```python
from build123d import *

# Parameters (mm, degrees)
SKETCH1_W              = 44
SKETCH1_H              = 26
BOSS_EXTRUDE1_DEPTH    = 1.45
SKETCH3_R              = 4
CUT_EXTRUDE1_DEPTH     = 52.128294515
SKETCH4_R              = 1
CUT_EXTRUDE2_DEPTH     = 52.128294515
CIRPATTERN1_COUNT      = 8
SKETCH7_R              = 1.25
CUT_EXTRUDE3_DEPTH     = 52.128294515
CIRPATTERN2_COUNT      = 8
SKETCH9_R              = 1.25
CUT_EXTRUDE4_DEPTH     = 52.128294515
CIRPATTERN3_COUNT      = 4
SKETCH10_R             = 1.25
CUT_EXTRUDE5_DEPTH     = 52.128294515
SKETCH11_R             = 1.25
CUT_EXTRUDE6_DEPTH     = 52.128294515
SKETCH14_W             = 4.5
SKETCH14_H             = 8
CUT_EXTRUDE7_DEPTH     = 52.128294515
FILLET1_R              = 1
FILLET1_OF_MIRROR2_R   = 1
SKETCH16_W             = 1.45
SKETCH16_H             = 26
BOSS_EXTRUDE4_DEPTH    = 31.05
SKETCH21_W             = 5
SKETCH21_H             = 8
CUT_EXTRUDE10_DEPTH    = 60.521025697
SKETCH22_R             = 4
CUT_EXTRUDE11_DEPTH    = 60.521025697
SKETCH23_R             = 1
CUT_EXTRUDE12_DEPTH    = 60.521025697
CIRPATTERN5_COUNT      = 8
SKETCH24_W             = 31.05
SKETCH24_H             = 2
CUT_EXTRUDE13_DEPTH    = 60.521025697
SKETCH26_W             = 31.05
SKETCH26_H             = 2
CUT_EXTRUDE14_DEPTH    = 60.521025697
FILLET3_R              = 2
SKETCH28_R             = 1
CUT_EXTRUDE16_DEPTH    = 10
SKETCH30_R             = 1
CUT_EXTRUDE17_DEPTH    = 10
SKETCH31_W             = 4
SKETCH31_H             = 10
CUT_EXTRUDE18_DEPTH    = 3
FILLET4_R              = 1
LPATTERN1_COUNT        = 2
LPATTERN1_PITCH        = 8
FILLET4_OF_LPATTERN1_R = 1
MIRROR3_START          = 42.55
MIRROR3_OUTLINE_R      = 1
MIRROR3_DEPTH          = 1.45
SKETCH34_W             = 39
SKETCH34_H             = 1.45
BOSS_EXTRUDE8_DEPTH    = 3.35
SKETCH37_W             = 2.5
SKETCH37_H             = 2
CUT_EXTRUDE20_DEPTH    = 3.35
SKETCH35_W             = 2.5
SKETCH35_H             = 2
CUT_EXTRUDE21_DEPTH    = 3.35
FILLET5_R              = 1.5
FILLET6_R              = 2
FILLET7_R              = 1.5
FILLET8_R              = 1.5
FILLET9_R              = 2


# Read off the part's stored shape, not the designer's step: Mirror3
with BuildPart() as part:
    # Sketch1 → Boss-Extrude1 (new body)
    with BuildSketch(Plane.XY):
        with Locations((22, 13)):
            Rectangle(SKETCH1_W, SKETCH1_H)
    extrude(amount=BOSS_EXTRUDE1_DEPTH)

    # Sketch3 → Cut-Extrude1 (cut, through all)
    with BuildSketch(Plane.XY.offset(1.45)):
        with Locations((22, 13)):
            Circle(SKETCH3_R)
    extrude(amount=-CUT_EXTRUDE1_DEPTH, mode=Mode.SUBTRACT)

    # Sketch4 → Cut-Extrude2 (cut, through all)
    with BuildSketch(Plane.XY.offset(1.45)):
        with Locations((22, 21)):
            Circle(SKETCH4_R)
    cut_extrude2 = extrude(amount=-CUT_EXTRUDE2_DEPTH, mode=Mode.SUBTRACT)

    # CirPattern1: Cut-Extrude2 ×8 about axis
    cirpattern1_axis = Axis((22, 13, 0), (0, 0, 1))
    for i in range(1, CIRPATTERN1_COUNT):
        add(cut_extrude2.rotate(cirpattern1_axis, i * 360 / CIRPATTERN1_COUNT), mode=Mode.SUBTRACT)

    # Sketch7 → Cut-Extrude3 (cut, through all)
    with BuildSketch(Plane.XY.offset(1.45)):
        with Locations((25.322496408, 21)):
            Circle(SKETCH7_R)
    cut_extrude3 = extrude(amount=-CUT_EXTRUDE3_DEPTH, mode=Mode.SUBTRACT)

    # CirPattern2: Cut-Extrude3 ×8 about axis
    cirpattern2_axis = Axis((22, 13, 0), (0, 0, 1))
    for i in range(1, CIRPATTERN2_COUNT):
        add(cut_extrude3.rotate(cirpattern2_axis, i * 360 / CIRPATTERN2_COUNT), mode=Mode.SUBTRACT)

    # Sketch9 → Cut-Extrude4 (cut, through all)
    with BuildSketch(Plane.XY.offset(1.45)):
        with Locations((30, 21)):
            Circle(SKETCH9_R)
    cut_extrude4 = extrude(amount=-CUT_EXTRUDE4_DEPTH, mode=Mode.SUBTRACT)

    # CirPattern3: Cut-Extrude4 ×4 about axis
    cirpattern3_axis = Axis((22, 13, 0), (0, 0, 1))
    for i in range(1, CIRPATTERN3_COUNT):
        add(cut_extrude4.rotate(cirpattern3_axis, i * 360 / CIRPATTERN3_COUNT), mode=Mode.SUBTRACT)

    # Sketch10 → Cut-Extrude5 (cut, through all)
    with BuildSketch(Plane.XY.offset(1.45)):
        with Locations((39.5, 21)):
            Circle(SKETCH10_R)
    cut_extrude5 = extrude(amount=-CUT_EXTRUDE5_DEPTH, mode=Mode.SUBTRACT)

    # Sketch11 → Cut-Extrude6 (cut, through all)
    with BuildSketch(Plane.XY.offset(1.45)):
        with Locations((39.5, 5)):
            Circle(SKETCH11_R)
    cut_extrude6 = extrude(amount=-CUT_EXTRUDE6_DEPTH, mode=Mode.SUBTRACT)

    # Mirror1: Cut-Extrude5, Cut-Extrude6 across plane
    add(cut_extrude5.mirror(Plane(origin=(22, 0, 0), x_dir=(0, 0, 1), z_dir=(1, 0, 0))), mode=Mode.SUBTRACT)
    add(cut_extrude6.mirror(Plane(origin=(22, 0, 0), x_dir=(0, 0, 1), z_dir=(1, 0, 0))), mode=Mode.SUBTRACT)

    # Sketch14 → Cut-Extrude7 (cut, through all)
    with BuildSketch(Plane.XY.offset(1.45)):
        with Locations((8.25, 13)):
            Rectangle(SKETCH14_W, SKETCH14_H)
    cut_extrude7 = extrude(amount=-CUT_EXTRUDE7_DEPTH, mode=Mode.SUBTRACT)

    # Fillet1
    fillet1_edges = [part.edges().sort_by_distance(p)[0] for p in [
        (10.5, 9, 0.725),
        (6, 9, 0.725),
        (6, 17, 0.725),
        (10.5, 17, 0.725),
    ]]
    fillet(fillet1_edges, radius=FILLET1_R)

    # Mirror2: Cut-Extrude7 across plane
    add(cut_extrude7.mirror(Plane(origin=(22, 0, 0), x_dir=(0, 0, 1), z_dir=(1, 0, 0))), mode=Mode.SUBTRACT)

    # Fillet1 of Mirror2
    fillet1_of_mirror2_edges = [part.edges().sort_by_distance(p)[0] for p in [
        (33.5, 9, 0.725),
        (38, 9, 0.725),
        (38, 17, 0.725),
        (33.5, 17, 0.725),
    ]]
    fillet(fillet1_of_mirror2_edges, radius=FILLET1_OF_MIRROR2_R)

    # Sketch16 → Boss-Extrude4 (add)
    with BuildSketch(Plane.XY.offset(1.45)):
        with Locations((0.725, 13)):
            Rectangle(SKETCH16_W, SKETCH16_H)
    extrude(amount=BOSS_EXTRUDE4_DEPTH)

    # Sketch21 → Cut-Extrude10 (cut, through all)
    with BuildSketch(Plane(origin=(1.45, 0, 0), x_dir=(0, 0, -1), z_dir=(1, 0, 0))):
        with Locations((-32.5, 13)):
            Rectangle(SKETCH21_W, SKETCH21_H)
    extrude(amount=-CUT_EXTRUDE10_DEPTH, mode=Mode.SUBTRACT)

    # Sketch22 → Cut-Extrude11 (cut, through all)
    with BuildSketch(Plane(origin=(1.45, 0, 0), x_dir=(0, 0, -1), z_dir=(1, 0, 0))):
        with Locations((-30, 13)):
            Circle(SKETCH22_R)
    extrude(amount=-CUT_EXTRUDE11_DEPTH, mode=Mode.SUBTRACT)

    # Sketch23 → Cut-Extrude12 (cut, through all)
    with BuildSketch(Plane(origin=(1.45, 0, 0), x_dir=(0, 0, -1), z_dir=(1, 0, 0))):
        with Locations((-22, 13)):
            Circle(SKETCH23_R)
    cut_extrude12 = extrude(amount=-CUT_EXTRUDE12_DEPTH, mode=Mode.SUBTRACT)

    # CirPattern5: Cut-Extrude12 ×8 about axis, 2 skipped
    cirpattern5_axis = Axis((0, 13, 30), (1, 0, 0))
    add([cut_extrude12.rotate(cirpattern5_axis, i * 360 / CIRPATTERN5_COUNT) for i in range(1, CIRPATTERN5_COUNT) if i not in (4, 5)], mode=Mode.SUBTRACT)

    # Sketch24 → Cut-Extrude13 (cut, through all)
    with BuildSketch(Plane(origin=(1.45, 0, 0), x_dir=(0, 0, -1), z_dir=(1, 0, 0))):
        with Locations((-16.975, 25)):
            Rectangle(SKETCH24_W, SKETCH24_H)
    extrude(amount=-CUT_EXTRUDE13_DEPTH, mode=Mode.SUBTRACT)

    # Sketch26 → Cut-Extrude14 (cut, through all)
    with BuildSketch(Plane(origin=(1.45, 0, 0), x_dir=(0, 0, -1), z_dir=(1, 0, 0))):
        with Locations((-16.975, 1)):
            Rectangle(SKETCH26_W, SKETCH26_H)
    extrude(amount=-CUT_EXTRUDE14_DEPTH, mode=Mode.SUBTRACT)

    # Fillet3
    fillet3_edges = [part.edges().sort_by_distance(p)[0] for p in [
        (0.725, 17, 32.5),
        (0.725, 9, 32.5),
        (0.725, 24, 32.5),
        (0.725, 2, 32.5),
    ]]
    fillet(fillet3_edges, radius=FILLET3_R)

    # Sketch28 → Cut-Extrude16 (cut)
    with BuildSketch(Plane.ZY):
        with Locations((12, 21)):
            Circle(SKETCH28_R)
    extrude(amount=-CUT_EXTRUDE16_DEPTH, mode=Mode.SUBTRACT)

    # Sketch30 → Cut-Extrude17 (cut)
    with BuildSketch(Plane.ZY):
        with Locations((12, 5)):
            Circle(SKETCH30_R)
    extrude(amount=-CUT_EXTRUDE17_DEPTH, mode=Mode.SUBTRACT)

    # Sketch31 → Cut-Extrude18 (cut)
    with BuildSketch(Plane.ZY):
        with Locations((16, 13)):
            Rectangle(SKETCH31_W, SKETCH31_H)
    cut_extrude18 = extrude(amount=-CUT_EXTRUDE18_DEPTH, mode=Mode.SUBTRACT)

    # Fillet4
    fillet4_edges = [part.edges().sort_by_distance(p)[0] for p in [
        (0.725, 8, 14),
        (0.725, 18, 14),
        (0.725, 18, 18),
        (0.725, 8, 18),
    ]]
    fillet(fillet4_edges, radius=FILLET4_R)

    # LPattern1: Cut-Extrude18 ×2
    with Locations(*[(0, 0, -i * LPATTERN1_PITCH) for i in range(1, LPATTERN1_COUNT)]):
        add(cut_extrude18, mode=Mode.SUBTRACT)

    # Fillet4 of LPattern1
    fillet4_of_lpattern1_edges = [part.edges().sort_by_distance(p)[0] for p in [
        (0.725, 8, 6),
        (0.725, 18, 6),
        (0.725, 18, 10),
        (0.725, 8, 10),
    ]]
    fillet(fillet4_of_lpattern1_edges, radius=FILLET4_OF_LPATTERN1_R)

    # Mirror3 outline → Mirror3 (add)
    with BuildSketch(Plane.YZ.offset(MIRROR3_START)):
        with BuildLine():
            Line((7, 32.5), (4, 32.5))
            ThreePointArc((4, 32.5), (2.585786438, 31.914213562), (2, 30.5))
            Line((2, 30.5), (2, 1.45))
            Line((2, 1.45), (24, 1.45))
            Line((24, 1.45), (24, 30.5))
            ThreePointArc((24, 30.5), (23.414213562, 31.914213562), (22, 32.5))
            Line((22, 32.5), (19, 32.5))
            ThreePointArc((19, 32.5), (17.585786438, 31.914213562), (17, 30.5))
            Line((17, 30.5), (17, 30))
            ThreePointArc((17, 30), (13, 26), (9, 30))
            Line((9, 30), (9, 30.5))
            ThreePointArc((9, 30.5), (8.414213562, 31.914213562), (7, 32.5))
        make_face()
        with Locations((5, 12)):
            Circle(MIRROR3_OUTLINE_R, mode=Mode.SUBTRACT)
        with BuildLine():
            Line((18, 9), (18, 7))
            ThreePointArc((18, 7), (17.707106781, 6.292893219), (17, 6))
            Line((17, 6), (9, 6))
            ThreePointArc((9, 6), (8.292893219, 6.292893219), (8, 7))
            Line((8, 7), (8, 9))
            ThreePointArc((8, 9), (8.292893219, 9.707106781), (9, 10))
            Line((9, 10), (17, 10))
            ThreePointArc((17, 10), (17.707106781, 9.707106781), (18, 9))
        make_face(mode=Mode.SUBTRACT)
        with BuildLine():
            ThreePointArc((18, 15), (17.707106781, 14.292893219), (17, 14))
            Line((17, 14), (9, 14))
            ThreePointArc((9, 14), (8.292893219, 14.292893219), (8, 15))
            Line((8, 15), (8, 17))
            ThreePointArc((8, 17), (8.292893219, 17.707106781), (9, 18))
            Line((9, 18), (17, 18))
            ThreePointArc((17, 18), (17.707106781, 17.707106781), (18, 17))
            Line((18, 17), (18, 15))
        make_face(mode=Mode.SUBTRACT)
        with Locations((21, 12)):
            Circle(MIRROR3_OUTLINE_R, mode=Mode.SUBTRACT)
        with Locations((7.343145751, 24.343145751)):
            Circle(MIRROR3_OUTLINE_R, mode=Mode.SUBTRACT)
        with Locations((5, 30)):
            Circle(MIRROR3_OUTLINE_R, mode=Mode.SUBTRACT)
        with Locations((13, 22)):
            Circle(MIRROR3_OUTLINE_R, mode=Mode.SUBTRACT)
        with Locations((18.656854249, 24.343145751)):
            Circle(MIRROR3_OUTLINE_R, mode=Mode.SUBTRACT)
        with Locations((21, 30)):
            Circle(MIRROR3_OUTLINE_R, mode=Mode.SUBTRACT)
    extrude(amount=MIRROR3_DEPTH)

    # Sketch34 → Boss-Extrude8 (add)
    with BuildSketch(Plane.XY.offset(1.45)):
        with Locations((22, 25.275)):
            Rectangle(SKETCH34_W, SKETCH34_H)
    boss_extrude8 = extrude(amount=BOSS_EXTRUDE8_DEPTH)

    # Sketch37 → Cut-Extrude20 (cut)
    with BuildSketch(Plane.XY.offset(1.45)):
        with Locations((42.75, 25)):
            Rectangle(SKETCH37_W, SKETCH37_H)
    cut_extrude20 = extrude(amount=-CUT_EXTRUDE20_DEPTH, mode=Mode.SUBTRACT)

    # Sketch35 → Cut-Extrude21 (cut)
    with BuildSketch(Plane.XY.offset(1.45)):
        with Locations((1.25, 25)):
            Rectangle(SKETCH35_W, SKETCH35_H)
    cut_extrude21 = extrude(amount=-CUT_EXTRUDE21_DEPTH, mode=Mode.SUBTRACT)

    # Fillet5
    fillet5_edges = [part.edges().sort_by_distance(p)[0] for p in [
        (22, 26, 0),
    ]]
    fillet(fillet5_edges, radius=FILLET5_R)

    # Fillet6
    fillet6_edges = [part.edges().sort_by_distance(p)[0] for p in [
        (2.5, 25.275, 4.8),
        (41.5, 25.275, 4.8),
    ]]
    fillet(fillet6_edges, radius=FILLET6_R)

    # Fillet7
    fillet7_edges = [part.edges().sort_by_distance(p)[0] for p in [
        (44, 12, 0),
        (0, 12, 0),
    ]]
    fillet(fillet7_edges, radius=FILLET7_R)

    # Mirror5: Boss-Extrude8, Cut-Extrude20, Cut-Extrude21 across plane
    add(boss_extrude8.mirror(Plane.ZX.offset(13)))
    add(cut_extrude20.mirror(Plane.ZX.offset(13)), mode=Mode.SUBTRACT)
    add(cut_extrude21.mirror(Plane.ZX.offset(13)), mode=Mode.SUBTRACT)

    # Fillet8
    fillet8_edges = [part.edges().sort_by_distance(p)[0] for p in [
        (22, 0, 0),
    ]]
    fillet(fillet8_edges, radius=FILLET8_R)

    # Fillet9
    fillet9_edges = [part.edges().sort_by_distance(p)[0] for p in [
        (2.5, 0.725, 4.8),
        (41.5, 0.725, 4.8),
    ]]
    fillet(fillet9_edges, radius=FILLET9_R)


solid = part.part
```
CAD build for the part. Positions are in the model's coordinates, mm. A direction names the side the tool comes from. Coordinates: 2 decimals unless noted, no trailing zeros. Order: outer loops, then holes, each group sorted by start corner. A loop starts at its lowest first (then second) coordinate and runs counter-clockwise, first axis right, second up. Notation, with made-up numbers: (4.25, -5.5) - (16.25, -5.5) arc R28 cw to (16.25, 21.5) - close; hole circle Ø6 at (29.5, -5.5). An arc over 180 degrees is marked (long way). Use a Markdown table: item, result. Add a question column.
(1) Saw through at B-B (x = 20.5). Give the cut face in (y, z), then the cut area to 3 significant figures.
(2) Saw through at C-C (y = 13). Count the separate pieces of the cut face and the enclosed holes in it, then the cut area to 3 significant figures.
(3) Pull direction Y, two halves, no side cores. Call faces 6 (the face through (0.735, 8.342, 24.386)), 7 (the face through (0, 13, 13)): +Y half, -Y half, draft (parallel to the pull), parting line (faces both ways), or undercut.
(4) Saw through at A-A (z = 22). Give the cut face in (x, y).
(5) Flat gauge pins, fed straight in: pin 1 (4 mm diameter, centred on x = 4.5, y = 21, fed in from +Z); pin 2 (3 mm diameter, centred on x = 30.01, y = 16.31, fed in from +Z); pin 3 (0.7 mm diameter, centred on x = 43.5, z = 16, fed in from +Y). Where does each tip first touch, or does it go through?
(6) Saw through at D-D (x = 11.5). Give the cut face in (y, z).
(7) Drill centre lines: line 1 along X through (y, z) = (10, 4.5); line 2 along Z through (x, y) = (43.7, 21); line 3 along Y through (x, z) = (28.5, 1). Where is each one in solid material? Low to high. Write a range as [from, to].
(8) Which spindle directions (+Z, -Z, +X, -X, +Y, -Y) get a long thin tool onto all of the face, cutting with end or side? Do faces 1 (the face through (22, 1, 4.8)), 2 (the face through (43.265, 8.285, 9.699)), 3 (the face through (17, 13, 0)), 4 (the face through (22, 1.45, 3)), 5 (the face through (36, 9, 1)). Say none if no direction does.
Solved:
| question | item | result |
|---|---|---|
| 1 | outline | (0, 1.5) arc R1.5 ccw to (1.5, 0) - (9.29, 0) - (9.29, 1.45) - (1.45, 1.45) - (1.45, 4.8) - (0, 4.8) - close; (16.71, 0) - (24.5, 0) arc R1.5 ccw to (26, 1.5) - (26, 4.8) - (24.55, 4.8) - (24.55, 1.45) - (16.71, 1.45) - close |
| 1 | area | 35.7 mm² |
| 2 | separate pieces | 12 |
| 2 | enclosed holes | 0 |
| 2 | area | 74.6 mm² |
| 3 | face 6 | undercut |
| 3 | face 7 | draft |
| 4 | outline | (0, 2) - (1.45, 2) - (1.45, 12) - (0, 12) - close; (0, 14) - (1.45, 14) - (1.45, 24) - (0, 24) - close; (42.55, 2) - (44, 2) - (44, 12) - (42.55, 12) - close; (42.55, 14) - (44, 14) - (44, 24) - (42.55, 24) - close |
| 5 | pin 1 | stops at z = 1.45 |
| 5 | pin 2 | stops at z = 1.45 |
| 5 | pin 3 | stops at y = 24 |
| 6 | outline | (0, 1.5) arc R1.5 ccw to (1.5, 0) - (24.5, 0) arc R1.5 ccw to (26, 1.5) - (26, 4.8) - (24.55, 4.8) - (24.55, 1.45) - (1.45, 1.45) - (1.45, 4.8) - (0, 4.8) - close |
| 7 | line 1 | x = [0, 1.45], [42.55, 44] |
| 7 | line 2 | z = [0.6, 11], [13, 29], [31, 32.5] |
| 7 | line 3 | y = [0.09, 6.81], [7.88, 18.12], [19.19, 25.91] |
| 8 | face 1 | +Z, +X, -X, +Y, -Y |
| 8 | face 2 | +X, -X |
| 8 | face 3 | -Z, +X, -X, +Y, -Y |
| 8 | face 4 | +Z, +X, -X |
| 8 | face 5 | +Z, -Z |
